Could you check a few things on this model? Use its own coordinates, in mm. A direction names the side the tool comes from. Round coordinates to 2 decimals unless told otherwise and drop trailing zeros. Loops run counter-clockwise (first coordinate to the right, second up) from the corner with the lowest first, then second, coordinate; pieces in that order, holes last.
from build123d import *

# Parameters (mm, degrees)
F1_DEPTH = 63.5
F0_W     = 25.4
F0_H     = 19.05
F2_DEPTH = 25.4
F3_DEPTH = 7.9375
F5_R     = 6.35


with BuildPart() as f1:
    # F0 (on Front) → F1 (new body, symmetric)
    with BuildSketch(Plane.XZ):
        Polygon((-41.275, 9.525), (-41.275, -9.525), (41.275, -9.525), (41.275, 9.525), (22.225, 9.525), align=None)
    extrude(amount=F1_DEPTH, both=True)

    # F0 (on Front) → F2 (join, symmetric)
    with BuildSketch(Plane.XZ):
        with BuildLine():
            Line((22.225, 9.525), (41.275, 9.525))
            Line((41.275, 9.525), (41.275, 27.0002))
            ThreePointArc((41.275, 27.0002), (45.92468, 38.22552), (57.15, 42.8752))
            Line((57.15, 42.8752), (60.325, 42.8752))
            Line((60.325, 42.8752), (60.325, 61.9252))
            Line((60.325, 61.9252), (57.15, 61.9252))
            ThreePointArc((57.15, 61.9252), (53.137152, 61.693898), (49.177457, 61.003056))
            add(Edge.make_bspline(
                [(36.107399, 54.874284), (40.299297, 57.685987), (44.600471, 59.850046), (49.177457, 61.003056)],
                knots=[85.334769, 85.334769, 85.334769, 85.334769, 102.114273, 102.114273, 102.114273, 102.114273], degree=3))
            ThreePointArc((36.107399, 54.874284), (25.887655, 42.570087), (22.225, 27.0002))
            Line((22.225, 27.0002), (22.225, 9.525))
        make_face()
        with Locations((73.025, 52.4002)):
            Rectangle(F0_W, F0_H)
    extrude(amount=F2_DEPTH, both=True)

    # F0 (on Front) → F3 (join, symmetric)
    with BuildSketch(Plane.XZ):
        with BuildLine():
            add(Edge.make_bspline(
                [(-41.275, 9.525), (-3.70342, 9.525), (14.788851, 40.574934), (36.107399, 54.874284)],
                knots=[0, 0, 0, 0, 85.334769, 85.334769, 85.334769, 85.334769], degree=3))
            Line((-41.275, 9.525), (22.225, 9.525))
            Line((22.225, 9.525), (22.225, 27.0002))
            ThreePointArc((22.225, 27.0002), (25.887655, 42.570087), (36.107399, 54.874284))
        make_face()
    extrude(amount=F3_DEPTH, both=True)

    # F0 (on Front) → F4 (revolve)
    with BuildSketch(Plane.XZ):
        Polygon((85.725, 61.9252), (85.725, 42.8752), (85.725, 38.1), (111.125, 38.1), (111.125, 66.675), (85.725, 66.675), align=None)
    revolve(axis=Axis((85.725, 0, 52.4002), (0, 0, 1)))

    # F5
    f5_edges = [f1.edges().sort_by_distance(p)[0] for p in [
        (-41.275, -63.5, 0),
        (41.275, -63.5, 0),
        (-41.275, 63.5, 0),
        (41.275, 63.5, 0),
    ]]
    fillet(f5_edges, radius=F5_R)


solid = f1.part
Item 1: Will these pins go through, and if not, where does the flat tip stop? pin 1 (2 mm diameter, centred on x = 18, y = -49, fed in from +Z) (3 decimals); pin 2 (1 mm diameter, centred on x = 71, y = -3, fed in from -Z); pin 3 (1.5 mm diameter, centred on x = 24, z = 39.5, fed in from +Y).
Results list:
pin 1: stops at z = 9.525
pin 2: stops at z = 38.1
pin 3: stops at y = 25.4
Item 2: If we section it at C-C, the plane x = 89.5: Please give me the cut outline in (y, z) (3 decimals).
Results list:
outline: (-25.118, 38.1) - (25.118, 38.1) - (25.118, 66.675) - (-25.118, 66.675) - close
Item 3: For faces 1 (the flat face through (60, -2, 61.925)), 2 (the flat face through (60, 2, 42.875)), 3 (the flat face through (46, -25.4, 42)), which set-ups out of +Z, -Z, +X, -X, +Y, -Y let a thin tool reach every point of the face, with its end or its side?
Results list:
face 1: +Z, -X
face 2: -Z
face 3: +Z, +X, -X, -Y
Item 4: If I drill on line 1 along X through (y, z) = (1, 8) (3 decimals); line 2 along Z through (x, y) = (38, 35.5) (3 decimals); line 3 along Y through (x, z) = (43.5, 37), over which ranges is the centre line in solid material (lowest first)?
Results list:
line 1: x = -41.275 to 41.275
line 2: z = -9.525 to 9.525
line 3: y = -25.4 to 25.4
Item 5: If we section it at A-A, the plane z = -3: Please give me the cut outline in (x, y) (3 decimals), then the cut area to 3 significant figures.
Results list:
outline: (-41.275, -57.15) arc R6.35 ccw to (-34.925, -63.5) - (34.925, -63.5) arc R6.35 ccw to (41.275, -57.15) - (41.275, 57.15) arc R6.35 ccw to (34.925, 63.5) - (-34.925, 63.5) arc R6.35 ccw to (-41.275, 57.15) - close
area: 10,400 mm2
Item 6: If we section it at B-B, the plane y = -39: Please give me the cut outline in (x, z) (3 decimals).
Results list:
outline: (-41.275, -9.525) - (41.275, -9.525) - (41.275, 9.525) - (-41.275, 9.525) - close
Item 7: We'd pull the mould along X, two halves only. Please class faces 4 (the cylindrical face through (25.99, -16.79, 42.77)), 5 (the flat face through (0, -63.5, 0)), 6 (the cylindrical face through (45.8, -0.4, 38.1)): released by +X, released by -X, zero draft, split by the parting line, or undercut.
Results list:
face 4: released by -X
face 5: zero draft
face 6: undercut
